from build123d import *

# Parameters (mm, degrees)
SKETCH1_R           = 38.1
BOSS_EXTRUDE1_DEPTH = 25.4
CUT_EXTRUDE1_DEPTH  = 6.35
CUT_EXTRUDE2_START  = -12.7
CUT_EXTRUDE2_DEPTH  = 12.7


with BuildPart() as part:
    # Sketch1 → Boss-Extrude1 (new body)
    with BuildSketch(Plane.XY):
        with BuildLine():
            Line((-41.275, -41.275), (-41.275, 41.275))
            Line((-41.275, 41.275), (0, 41.275))
            Line((0, 41.275), (0, 47.625))
            ThreePointArc((0, 47.625), (47.625, 0), (0, -47.625))
            Line((0, -47.625), (0, -41.275))
            Line((0, -41.275), (-41.275, -41.275))
        make_face()
        Circle(SKETCH1_R, mode=Mode.SUBTRACT)
    extrude(amount=BOSS_EXTRUDE1_DEPTH)

    # Sketch5 → Cut-Revolve3 (revolve, cut)
    with BuildSketch(Plane(origin=(0, 0, 12.7), x_dir=(-1, 0, 0), z_dir=(0, 0, -1))):
        with BuildLine():
            Line((0.422989948, -1.197488832), (-13.958668291, 39.517131469))
            ThreePointArc((-13.958668291, 39.517131469), (-27.125149322, 11.968992199), (0.422989948, -1.197488832))
        make_face()
    revolve(axis=Axis((-0.422989948, -1.197488832, 12.7), (0.333062951, 0.942904592, 0)), mode=Mode.SUBTRACT)

    # Sketch2 → Cut-Extrude1 (cut)
    with BuildSketch(Plane.XY.offset(25.4)):
        with BuildLine():
            Line((-6.286105585, 39.186509577), (0, 0))
            Line((0, 0), (28.956627522, 27.140585455))
            ThreePointArc((28.956627522, 27.140585455), (-12.836051309, -37.55440644), (-6.286105585, 39.186509577))
        make_face()
    extrude(amount=-CUT_EXTRUDE1_DEPTH, mode=Mode.SUBTRACT)

    # Sketch4 → Cut-Extrude2 (cut)
    with BuildSketch(Plane(origin=(0, 0, 0), x_dir=(-1, 0, 0), z_dir=(0, 0, -1)).offset(CUT_EXTRUDE2_START)):
        with BuildLine():
            Line((0, 38.1), (0, -41.275))
            Line((0, -41.275), (41.275, -41.275))
            Line((41.275, -41.275), (41.275, 41.275))
            ThreePointArc((41.275, 41.275), (20.706704521, 38.787841223), (0, 38.1))
        make_face()
    extrude(amount=CUT_EXTRUDE2_DEPTH, mode=Mode.SUBTRACT)


solid = part.part
Work out the finished part from the listing and answer in its coordinate system (mm). A direction names the side the tool comes from. Coordinates: 2 decimals unless noted, no trailing zeros. Loops run counter-clockwise (first coordinate to the right, second up) from the corner with the lowest first, then second, coordinate; pieces in that order, holes last. Notation, with made-up numbers: M 40.5,53 L 65.5,53 A26 cw 65.5,89 Z; hole C 58,78 d5. An arc over 180 degrees is marked long. Answer in a Markdown table with one row per item. Add a question column.
1. Find section D-D, the plane z = 2.75. Write down the section's boundary in (x, y) (3 decimals), then the cut area to 3 significant figures.
2. Consider L1, parallel to X at y = 0, z = 23.25 (1 decimal); L2, parallel to X at y = -0.5, z = 19 (3 decimals); L3, parallel to X at y = 0, z = 10 (3 decimals). Determine where each line is inside the solid, lowest interval first.
3. Flat-ended cylindrical pins translate along their axes: P1, Ø12, axis at y = -35.5, z = 13.5, coming from the +X side; P2, Ø1.5, axis at y = 29, z = 10, coming from the -X side; P3, Ø4, axis at x = 18, z = 8.5, coming from the +Y side. Find the tip coordinate at first contact, or state that the pin passes through.
4. A tool of negligible diameter and unlimited length cuts with its end or side. For faces 1 (the cylindrical face through (-11.433, -38.005, 22.269)), 2 (the flat face through (-41.275, -1, 19)), 3 (the flat face through (40, 4, 25.4)), 4 (the flat face through (-39, -6, 12.7)), 5 (the flat face through (-21, 41.275, 13)), from which of +Z, -Z, +X, -X, +Y, -Y can it reach the whole face along a straight path? Write none if from no direction.
5. The mould has two halves that part along Y. Classify faces 6 (the flat face through (6, -38, 19.05)), 7 (the cylindrical face through (47.613, 1.047, 12.522)), 8 (the flat face through (-20, -41.275, 19)): pulls with the +Y half, pulls with the -Y half, needs draft (parallel to the pull), parting line crosses it, or undercut.
6. Find section C-C, the plane y = 13. Write down the section's boundary in (x, z) (3 decimals), then the cut area to 3 significant figures.
Reported:
| question | item | result |
|---|---|---|
| 1 | outline | M -41.275,41.275 A237.855 ccw -0.68,38.094 A38.1 cw 3.128,37.971 A19.161 cw 21.416,31.512 A38.1 cw 0,-38.1 L 0,-47.625 A47.625 ccw 0,47.625 L 0,41.275 Z |
| 1 | area | 1,350 mm^2 |
| 2 | L1 | x = -41.3 to -39.7, 39.7 to 47.6 |
| 2 | L2 | x = -41.275 to -38.097, 38.097 to 47.622 |
| 2 | L3 | x = 38.1 to 47.625 |
| 3 | P1 | stops at x = 37.39 |
| 3 | P2 | stops at x = 25.37 |
| 3 | P3 | stops at y = 44.86 |
| 4 | face 1 | +Z |
| 4 | face 2 | +Z, -Z, -X, +Y, -Y |
| 4 | face 3 | +Z, +X, -X, +Y, -Y |
| 4 | face 4 | -Z, -X, -Y |
| 4 | face 5 | +Z, -Z, -X, +Y |
| 5 | face 6 | undercut |
| 5 | face 7 | parting line crosses it |
| 5 | face 8 | pulls with the -Y half |
| 6 | outline | M -41.275,12.7 L -35.814,12.7 L -35.814,19.05 L -37.498,19.05 L -37.498,25.4 L -41.275,25.4 Z; M 35.814,0 L 45.816,0 L 45.816,25.4 L 37.498,25.4 L 37.498,19.05 L 35.814,19.05 Z |
| 6 | area | 302 mm^2 |
